from build123d import *

# Parameters (mm, degrees)
BOSS_EXTRUDE1_DEPTH      = 317.499999
BOSS_EXTRUDE1_DEPTH_BACK = 317.499999
SKETCH3_W                = 38.1
SKETCH3_H                = 25.4
SKETCH3_W_2              = 31.75
SKETCH3_H_2              = 19.05
F_10_CLEARANCE_HOLE2_D   = 4.9784
F_10_CLEARANCE_HOLE4_D   = 4.9784
F_10_CLEARANCE_HOLE3_D   = 4.9784


with BuildPart() as part:
    # Sketch3 → Boss-Extrude1 (new, two sides: drawn at the far end of the back side and taken through both)
    with BuildSketch(Plane.XY.offset(-BOSS_EXTRUDE1_DEPTH_BACK)):
        Rectangle(SKETCH3_W, SKETCH3_H)
        Rectangle(SKETCH3_W_2, SKETCH3_H_2, mode=Mode.SUBTRACT)
    extrude(amount=BOSS_EXTRUDE1_DEPTH + BOSS_EXTRUDE1_DEPTH_BACK)

    # #10 Clearance Hole2 (through all)
    with Locations(Plane.ZY.offset(19.05)):
        with Locations((-304.800000508, 0), (-279.400000508, 0), (279.399999492, 0), (304.799999492, 0)):
            Hole(F_10_CLEARANCE_HOLE2_D / 2)

    # #10 Clearance Hole4 (through all)
    with Locations(Plane(origin=(19.05, 0, 0), x_dir=(0, 0, -1), z_dir=(1, 0, 0))):
        with Locations((-252.857000506, 8e-09), (-227.457000506, 1.1e-08), (-124.587000507, 1.943404818), (-99.187000507, 1.943404821)):
            Hole(F_10_CLEARANCE_HOLE4_D / 2)

    # #10 Clearance Hole3 (through all)
    with Locations(Plane.ZY.offset(19.05)):
        with Locations((-50.8, 0), (50.8, 0)):
            Hole(F_10_CLEARANCE_HOLE3_D / 2)


solid = part.part
Model file for the job. Use its own axes, mm. A direction names the side the tool comes from. Give positions to 0.01 mm unless a question says otherwise; leave off trailing zeros. Order: outer loops, then holes, each group sorted by start corner. A loop starts at its lowest first (then second) coordinate and runs counter-clockwise, first axis right, second up. Notation, with made-up numbers: M -2,69 L 19,69 A7 ccw 19,81 Z; hole C -20.5,48 d8. An arc over 180 degrees is marked long. Write item = value, one per line.
Q1. Two-plate mould, pull along X, no slides. Class faces 3 (the flat face through (-19.05, 0, -4)), 4 (the flat face through (-15.875, 0, -4)), 5 (the flat face through (19.05, 0, -4)): pulls with the +X half, pulls with the -X half, needs draft (parallel to the pull), parting line crosses it, or undercut.
Derived:
face_3 = pulls with the -X half
face_4 = undercut
face_5 = pulls with the +X half
Q2. Tool access for faces 1 (the flat face through (0, 9.525, -4)), 2 (the flat face through (0, -11, -317.5)): list every direction of +Z, -Z, +X, -X, +Y, -Y with a clear straight run to the whole face (end or side of a thin tool).
Derived:
face_1 = +Z, -Z
face_2 = -Z, +X, -X, +Y, -Y
Q3. Cut at A-A, the plane x = -2.5. List the corners of the cut face in (y, z) (3 decimals).
Derived:
outline = M -12.7,-317.5 L -9.525,-317.5 L -9.525,317.5 L -12.7,317.5 Z; M 9.525,-317.5 L 12.7,-317.5 L 12.7,317.5 L 9.525,317.5 Z
Q4. Cut at B-B, the plane z = -78.5. List the corners of the cut face in (x, y) (3 decimals).
Derived:
outline = M -19.05,-12.7 L 19.05,-12.7 L 19.05,12.7 L -19.05,12.7 Z; hole M -15.875,-9.525 L 15.875,-9.525 L 15.875,9.525 L -15.875,9.525 Z
Q5. Drill centre lines: line 1 (X direction, y = 5.75, z = -110.5) (3 decimals); line 2 (Y direction, x = -14.5, z = -253.5) (3 decimals). Where is each one in solid material? Low to high. Write a range as [from, to].
Derived:
line_1 = [-19.05, -15.875], [15.875, 19.05]
line_2 = [-12.7, -9.525], [9.525, 12.7]
